from build123d import *

# Parameters (mm, degrees)
F0_R      = 25.4
F0_R_2    = 12.7
F1_DEPTH  = 50.8
F3_DEPTH  = 12.7
F5_DEPTH  = 12.7
F8_DEPTH  = 25.4
F10_DEPTH = 12.7


with BuildPart() as f1:
    # F0 (on Right) → F1 (new body)
    with BuildSketch(Plane.YZ):
        Circle(F0_R)
        Circle(F0_R_2, mode=Mode.SUBTRACT)
    extrude(amount=F1_DEPTH)

    # F2 (on face) → F3 (join)
    with BuildSketch(Plane.YZ.offset(50.8)):
        with BuildLine():
            Line((-8.40026, -9.525), (-23.54643, -9.525))
            ThreePointArc((-23.54643, -9.525), (0, -25.4), (23.54643, -9.525))
            Line((23.54643, -9.525), (8.40026, -9.525))
            ThreePointArc((8.40026, -9.525), (0, -12.7), (-8.40026, -9.525))
        make_face()
    extrude(amount=F3_DEPTH)

    # F4 (on face) → F5 (join)
    with BuildSketch(Plane.YZ.offset(63.5)):
        with BuildLine():
            ThreePointArc((-23.54643, -9.525), (0, -25.4), (23.54643, -9.525))
            ThreePointArc((23.54643, -9.525), (25.4, 0), (23.54643, 9.525))
            Line((23.54643, 9.525), (8.40026, 9.525))
            ThreePointArc((8.40026, 9.525), (12.7, 0), (8.40026, -9.525))
            ThreePointArc((8.40026, -9.525), (0, -12.7), (-8.40026, -9.525))
            ThreePointArc((-8.40026, -9.525), (-12.7, 0), (-8.40026, 9.525))
            Line((-8.40026, 9.525), (-23.54643, 9.525))
            ThreePointArc((-23.54643, 9.525), (-25.4, 0), (-23.54643, -9.525))
        make_face()
    extrude(amount=F5_DEPTH)

    # F7 (on offset) → F8 (join)
    with BuildSketch(Plane.XZ.offset(12.7)):
        Polygon((19.05, 25.4), (0, 25.4), (0, 19.05), (23.8125, 19.05), align=None)
        Polygon((0, 38.1), (0, 25.4), (19.05, 25.4), (9.525, 38.1), align=None)
    extrude(amount=-F8_DEPTH)

    # F9 (on face) → F10 (join)
    with BuildSketch(Plane(origin=(0, 12.7, 0), x_dir=(-1, 0, 0), z_dir=(0, 1, 0))):
        Polygon((0, 25.4), (0, 38.1), (-9.525, 38.1), (-38.1, 0), (0, 0), align=None)
        Polygon((-9.525, 38.1), (0, 38.1), (0, 50.8), align=None)
    extrude(amount=F10_DEPTH)


solid = f1.part
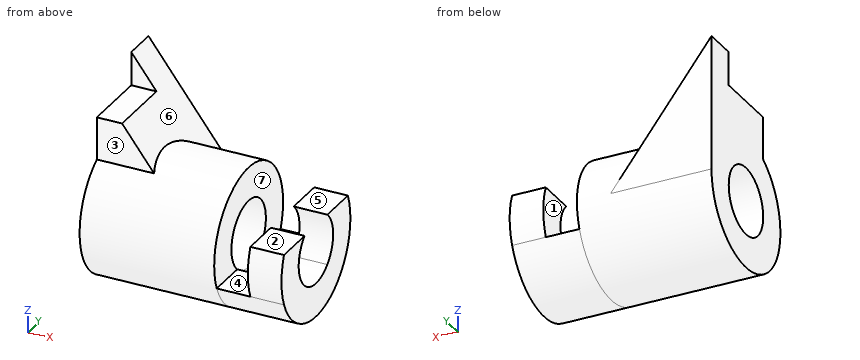
Work out the finished part from the listing and answer in its coordinate system (mm). Face numbers are marked on the shaded views. A direction names the side the tool comes from. Round coordinates to 2 decimals unless told otherwise and drop trailing zeros. Order: outer loops, then holes, each group sorted by start corner. A loop starts at its lowest first (then second) coordinate and runs counter-clockwise, first axis right, second up. Notation, with made-up numbers: M 67,36.5 L 94,36.5 A24 cw 94,72.5 Z; hole C 82,29.25 d4. An arc over 180 degrees is marked long. One line per item, written item: value.
Q1. Find section B-B on z = 11. Write down the section's boundary in (x, y).
Derived:
outline: M 0,-22.89 L 50.8,-22.89 L 50.8,-6.35 L 0,-6.35 Z; M 0,6.35 L 50.8,6.35 L 50.8,22.89 L 29.85,22.89 L 29.85,25.4 L 0,25.4 Z
Q2. Determine the mould class of the marked faces 4, 5, 6 and 7 for opening direction X: released by +X, released by -X, zero draft, split by the parting line, or undercut.
Derived:
face 4: undercut
face 5: zero draft
face 6: released by +X
face 7: undercut
Q3. Find section D-D on z = -1.5. Write down the section's boundary in (x, y), then the cut area to 3 significant figures.
Derived:
outline: M 0,-25.36 L 50.8,-25.36 L 50.8,-12.61 L 0,-12.61 Z; M 0,12.61 L 50.8,12.61 L 50.8,25.36 L 0,25.36 Z; M 63.5,-25.36 L 76.2,-25.36 L 76.2,-12.61 L 63.5,-12.61 Z; M 63.5,12.61 L 76.2,12.61 L 76.2,25.36 L 63.5,25.36 Z
area: 1,620 mm²
Q4. Flat-ended cylindrical pins translate along their axes: pin 1 (5 mm diameter, centred on x = 13.5, z = 27.5, fed in from -Y); pin 2 (3 mm diameter, centred on x = 4.5, z = 43.5, fed in from -Y); pin 3 (14 mm diameter, centred on x = 68.5, y = 19, fed in from +Z) (3 decimals); pin 4 (5 mm diameter, centred on y = -13.5, z = 2, fed in from -X). Find the tip coordinate at first contact, or state that the pin passes through.
Derived:
pin 1: y = -12.7
pin 2: y = 12.7
pin 3: z = 9.525
pin 4: x = 0
Q5. Find section A-A on y = 0. Write down the section's boundary in (x, z) (3 decimals).
Derived:
outline: M 0,-25.4 L 76.2,-25.4 L 76.2,-12.7 L 0,-12.7 Z; M 0,12.7 L 50.8,12.7 L 50.8,25.4 L 19.05,25.4 L 9.525,38.1 L 0,38.1 Z
Q6. Straight lines are drawn through the part: line 1 (Z direction, x = 29.5, y = 0); line 2 (Y direction, x = 29.5, z = 9). For each, find the intervals that lie inside material, in ascending order.
Derived:
line 1: -25.4 to -12.7, 12.7 to 25.4
line 2: -23.75 to -8.96, 8.96 to 25.4
Q7. For the marked faces 1, 2 and 3, determine the directions among +Z, -Z, +X, -X, +Y, -Y from which every point of the face is accessible in a straight line to the end or side of a thin tool.
Derived:
face 1: +Z, +Y, -Y
face 2: +Z, +X, +Y, -Y
face 3: +Z, +X, -X, -Y
Q8. Find section C-C on x = 65. Write down the section's boundary in (y, z) (3 decimals), then the cut area to 3 significant figures.
Derived:
outline: M -23.546,-9.525 A25.4 ccw 23.546,-9.525 A25.4 ccw 23.546,9.525 L 8.4,9.525 A12.7 cw 8.4,-9.525 A12.7 cw -8.4,-9.525 A12.7 cw -8.4,9.525 L -23.546,9.525 A25.4 ccw Z
area: 1,020 mm²
